The listing builds one solid part. Answer for the finished solid, in the listing's coordinates (mm). Face numbers are marked on the shaded views. A direction names the side the tool comes from. Coordinates: 2 decimals unless noted, no trailing zeros. Loops run counter-clockwise (first coordinate to the right, second up) from the corner with the lowest first, then second, coordinate; pieces in that order, holes last. Notation, with made-up numbers: (-37.75, -11.5) -> (17.25, -11.5) arc R20 ccw to (17.25, -5.5) -> close; hole circle Ø5 at (-8.75, 0). An arc over 180 degrees is marked (long way). Answer in a Markdown table with one row per item.
```python
from build123d import *

# Parameters (mm, degrees)
F0_W     = 25.8
F0_H     = 49.1
F0_W_2   = 24.2
F0_H_2   = 47.5
F1_DEPTH = 2
F2_W     = 25.8
F2_H     = 49.1
F2_W_2   = 24.2
F2_H_2   = 47.5
F3_DEPTH = 15
F4_W     = 21.8
F4_H     = 10.2
F5_DEPTH = 0.8
F6_W     = 10
F6_H     = 6
F7_DEPTH = 0.8


with BuildPart() as f1:
    # F0 (on Top) → F1 (new body)
    with BuildSketch(Plane.XY):
        Rectangle(F0_W, F0_H)
        Rectangle(F0_W_2, F0_H_2, mode=Mode.SUBTRACT)
        Rectangle(F0_W_2, F0_H_2)
    extrude(amount=F1_DEPTH)

    # F2 (on face) → F3 (join)
    with BuildSketch(Plane.XY.offset(2)):
        Rectangle(F2_W, F2_H)
        Rectangle(F2_W_2, F2_H_2, mode=Mode.SUBTRACT)
    extrude(amount=F3_DEPTH)

    # F4 (on face) → F5 (cut, through all)
    with BuildSketch(Plane.XZ.offset(24.55)):
        with Locations((0, 7.9)):
            Rectangle(F4_W, F4_H)
    extrude(amount=-F5_DEPTH, mode=Mode.SUBTRACT)

    # F6 (on face) → F7 (cut, through all)
    with BuildSketch(Plane(origin=(0, 24.55, 0), x_dir=(-1, 0, 0), z_dir=(0, 1, 0))):
        with Locations((-1.9, 8)):
            Rectangle(F6_W, F6_H)
    extrude(amount=-F7_DEPTH, mode=Mode.SUBTRACT)


solid = f1.part
```
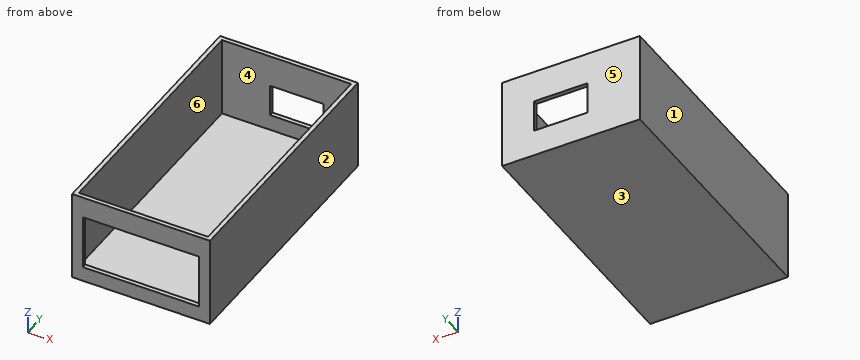
Item 1: A tool of negligible diameter and unlimited length cuts with its end or side. For the marked faces 5 and 6, from which of +Z, -Z, +X, -X, +Y, -Y can it reach the whole face along a straight path? Write none if from no direction.
Findings below:
| item | result |
|---|---|
| face 5 | +Z, -Z, +X, -X, +Y |
| face 6 | +Z |
Item 2: Determine the mould class of the marked faces 1, 2, 3 and 4 for opening direction X: +X half, -X half, draft (parallel to the pull), parting line (faces both ways), or undercut.
Findings below:
| item | result |
|---|---|
| face 1 | -X half |
| face 2 | +X half |
| face 3 | draft |
| face 4 | undercut |
Item 3: A cutting plane is placed at D-D, the plane x = -7.75. Determine the outline of the cut face in (y, z), plus the area to 3 significant figures.
Findings below:
| item | result |
|---|---|
| outline | (-24.55, 0) -> (24.55, 0) -> (24.55, 17) -> (23.75, 17) -> (23.75, 2) -> (-23.75, 2) -> (-23.75, 2.8) -> (-24.55, 2.8) -> close; (-24.55, 13) -> (-23.75, 13) -> (-23.75, 17) -> (-24.55, 17) -> close |
| area | 114 mm2 |
Item 4: Find the intervals of material crossed by probe 1 along Y at (x, z) = (10.75, 14.5); probe 2 along X at (y, z) = (23.5, 12.25); probe 3 along Y at (x, z) = (10.5, 4), in increasing order.
Findings below:
| item | result |
|---|---|
| probe 1 | y = -24.55 to -23.75, 23.75 to 24.55 |
| probe 2 | x = -12.9 to -12.1, 12.1 to 12.9 |
| probe 3 | y = 23.75 to 24.55 |
Item 5: A cutting plane is placed at A-A, the plane z = 15. Determine the outline of the cut face in (x, y).
Findings below:
| item | result |
|---|---|
| outline | (-12.9, -24.55) -> (12.9, -24.55) -> (12.9, 24.55) -> (-12.9, 24.55) -> close; hole (-12.1, -23.75) -> (12.1, -23.75) -> (12.1, 23.75) -> (-12.1, 23.75) -> close |
Item 6: A flat-ended cylindrical pin translates along its axis: pin 1 Ø7.5 at (x, y) = (1, -3.5) entering from +Z. Find the tip coordinate at first contact, or state that the pin passes through.
Findings below:
| item | result |
|---|---|
| pin 1 | stops at z = 2 |
Item 7: A cutting plane is placed at C-C, the plane z = 7.75. Determine the outline of the cut face in (x, y), plus the area to 3 significant figures.
Findings below:
| item | result |
|---|---|
| outline | (-12.9, -24.55) -> (-10.9, -24.55) -> (-10.9, -23.75) -> (-12.1, -23.75) -> (-12.1, 23.75) -> (-3.1, 23.75) -> (-3.1, 24.55) -> (-12.9, 24.55) -> close; (6.9, 23.75) -> (12.1, 23.75) -> (12.1, -23.75) -> (10.9, -23.75) -> (10.9, -24.55) -> (12.9, -24.55) -> (12.9, 24.55) -> (6.9, 24.55) -> close |
| area | 91.8 mm2 |
Item 8: A cutting plane is placed at B-B, the plane x = 2.75. Determine the outline of the cut face in (y, z), plus the area to 3 significant figures.
Findings below:
| item | result |
|---|---|
| outline | (-24.55, 0) -> (24.55, 0) -> (24.55, 5) -> (23.75, 5) -> (23.75, 2) -> (-23.75, 2) -> (-23.75, 2.8) -> (-24.55, 2.8) -> close; (-24.55, 13) -> (-23.75, 13) -> (-23.75, 17) -> (-24.55, 17) -> close; (23.75, 11) -> (24.55, 11) -> (24.55, 17) -> (23.75, 17) -> close |
| area | 109 mm2 |
